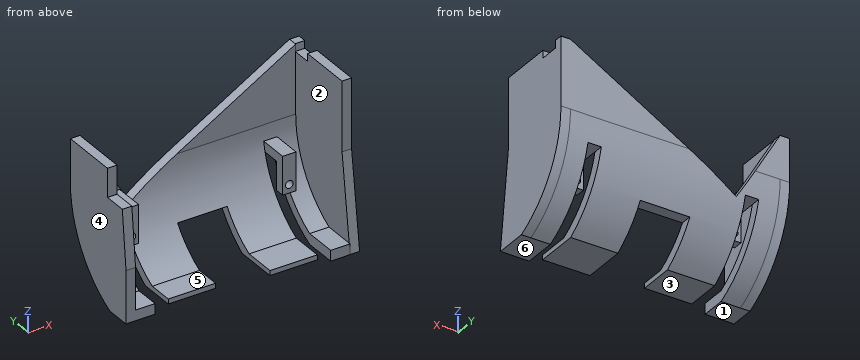
from build123d import *

# Parameters (mm, degrees)
BOSS_EXTRUDE1_DEPTH = 110
CUT_EXTRUDE1_DEPTH  = 110
SKETCH3_W           = 110
SKETCH3_H           = 22.912878475
CUT_EXTRUDE2_DEPTH  = 110
SKETCH4_W           = 10.2
SKETCH4_H           = 5.559027913
SKETCH4_W_2         = 24.8
SKETCH4_H_2         = 2.559027913
BOSS_EXTRUDE2_DEPTH = 13
SKETCH5_W           = 7
SKETCH5_H           = 5
BOSS_EXTRUDE3_DEPTH = 16
SKETCH6_W           = 10.2
SKETCH6_H           = 5.559027913
SKETCH6_W_2         = 24.8
SKETCH6_H_2         = 2.559027913
BOSS_EXTRUDE4_DEPTH = 4
CUT_EXTRUDE3_DEPTH  = 64
SKETCH8_W           = 7
SKETCH8_H           = 5
BOSS_EXTRUDE5_DEPTH = 15
SKETCH9_R           = 2
CUT_EXTRUDE4_DEPTH  = 10
BOSS_EXTRUDE6_START = 5
BOSS_EXTRUDE6_DEPTH = 5
BOSS_EXTRUDE7_DEPTH = 5


with BuildPart() as part:
    # Sketch1 → Boss-Extrude1 (new body)
    with BuildSketch(Plane(origin=(0, 0, 0), x_dir=(0, 0, -1), z_dir=(1, 0, 0))):
        with BuildLine():
            Line((0, 55), (-36, 55))
            Line((-36, 55), (-36, 50))
            Line((-36, 50), (0, 50))
            ThreePointArc((0, 50), (35.355339059, 35.355339059), (50, 0))
            Line((50, 0), (50, -1))
            Line((50, -1), (55, -1))
            Line((55, -1), (55, 0))
            ThreePointArc((55, 0), (38.890872965, 38.890872965), (0, 55))
        make_face()
    extrude(amount=BOSS_EXTRUDE1_DEPTH)

    # Sketch2 → Cut-Extrude1 (cut)
    with BuildSketch(Plane(origin=(0, 55, 0), x_dir=(1, 0, 0), z_dir=(0, 1, 0))):
        Polygon((99.8, 13), (92.8, 13), (92.8, 47), (68, 47), (68, 29), (42, 29), (42, 47), (17.2, 47), (17.2, 13), (10.2, 13), (10.2, 50), (-27.805612869, 50), (-27.805612869, 77.075699265), (114.223867828, 77.075699265), (114.223867828, 50), (99.8, 50), align=None)
    extrude(amount=-CUT_EXTRUDE1_DEPTH, mode=Mode.SUBTRACT)

    # Sketch3 → Cut-Extrude2 (cut)
    with BuildSketch(Plane(origin=(0, 0, -50), x_dir=(-1, 0, 0), z_dir=(0, 0, -1))):
        with Locations((-55, 11.456439238)):
            Rectangle(SKETCH3_W, SKETCH3_H)
    extrude(amount=-CUT_EXTRUDE2_DEPTH, mode=Mode.SUBTRACT)

    # Sketch4 → Boss-Extrude2 (add)
    with BuildSketch(Plane.XZ.offset(-22.912878475)):
        with Locations((104.9, -47.220486044)):
            Rectangle(SKETCH4_W, SKETCH4_H)
        with Locations((80.4, -45.720486044)):
            Rectangle(SKETCH4_W_2, SKETCH4_H_2)
        with Locations((29.6, -45.720486044)):
            Rectangle(SKETCH4_W_2, SKETCH4_H_2)
        with Locations((5.1, -47.220486044)):
            Rectangle(SKETCH4_W, SKETCH4_H)
    extrude(amount=BOSS_EXTRUDE2_DEPTH)

    # Sketch5 → Boss-Extrude3 (add)
    with BuildSketch(Plane.XZ.offset(-50)):
        with Locations((13.7, -10.5)):
            Rectangle(SKETCH5_W, SKETCH5_H)
        with Locations((96.3, -10.5)):
            Rectangle(SKETCH5_W, SKETCH5_H)
    extrude(amount=BOSS_EXTRUDE3_DEPTH)

    # Sketch6 → Boss-Extrude4 (add)
    with BuildSketch(Plane.XZ.offset(-9.912878475)):
        with Locations((104.9, -47.220486044)):
            Rectangle(SKETCH6_W, SKETCH6_H)
        with Locations((80.4, -45.720486044)):
            Rectangle(SKETCH6_W_2, SKETCH6_H_2)
    extrude(amount=BOSS_EXTRUDE4_DEPTH)

    # Sketch7 → Cut-Extrude3 (cut)
    with BuildSketch(Plane(origin=(0, 55, 0), x_dir=(1, 0, 0), z_dir=(0, 1, 0))):
        Polygon((110, -36), (21.665408814, 15), (0, -22.525588833), (0, -36), align=None)
    extrude(amount=-CUT_EXTRUDE3_DEPTH, mode=Mode.SUBTRACT)

    # Sketch8 → Boss-Extrude5 (add)
    with BuildSketch(Plane(origin=(0, 0, -13), x_dir=(-1, 0, 0), z_dir=(0, 0, -1))):
        with Locations((-13.7, 36.5)):
            Rectangle(SKETCH8_W, SKETCH8_H)
        with Locations((-96.3, 36.5)):
            Rectangle(SKETCH8_W, SKETCH8_H)
    extrude(amount=BOSS_EXTRUDE5_DEPTH)

    # Sketch9 → Cut-Extrude4 (cut)
    with BuildSketch(Plane(origin=(0, 39, 0), x_dir=(1, 0, 0), z_dir=(0, 1, 0))):
        with Locations(Location((13.7, 23.6, 0), (0, 0, 270))):
            Circle(SKETCH9_R)
        with Locations(Location((96.3, 23.6, 0), (0, 0, 270))):
            Circle(SKETCH9_R)
    extrude(amount=-CUT_EXTRUDE4_DEPTH, mode=Mode.SUBTRACT)

    # Sketch10 → Boss-Extrude6 (add)
    with BuildSketch(Plane.ZY.offset(BOSS_EXTRUDE6_START)):
        with BuildLine():
            Line((-50, 9.912878475), (-22.474411167, 9.912878475))
            Line((-22.474411167, 9.912878475), (7.525588833, 12.912878475))
            Line((7.525588833, 12.912878475), (7.525588833, 24.912878475))
            Line((7.525588833, 24.912878475), (22.525588833, 24.912878475))
            Line((22.525588833, 24.912878475), (22.525588833, 55))
            Line((22.525588833, 55), (0, 55))
            ThreePointArc((0, 55), (-29.705148408, 46.28827236), (-50, 22.912878475))
            Line((-50, 22.912878475), (-50, 9.912878475))
        make_face()
    extrude(amount=-BOSS_EXTRUDE6_DEPTH)

    # Sketch11 → Boss-Extrude7 (add)
    with BuildSketch(Plane(origin=(110, 0, 0), x_dir=(0, 0, -1), z_dir=(1, 0, 0))):
        with BuildLine():
            Line((-36, 50.412878475), (-32, 50.412878475))
            Line((-32, 50.412878475), (-32, 40.412878475))
            Line((-32, 40.412878475), (-36, 40.412878475))
            Line((-36, 40.412878475), (-36, 12.412878475))
            Line((-36, 12.412878475), (0.424300308, 12.412878475))
            Line((0.424300308, 12.412878475), (50, 5.912878475))
            Line((50, 5.912878475), (50, 22.912878475))
            ThreePointArc((50, 22.912878475), (29.705148408, 46.28827236), (0, 55))
            Line((0, 55), (-36, 55))
            Line((-36, 55), (-36, 50.412878475))
        make_face()
    extrude(amount=BOSS_EXTRUDE7_DEPTH)


solid = part.part
Read the model definition and answer for the solid it produces. Units are mm, in the model's axes. Face numbers are marked on the shaded views. A direction names the side the tool comes from. Give positions to 0.01 mm unless a question says otherwise; leave off trailing zeros. Write each loop counter-clockwise with the first axis right and the second up, starting at its lowest first coordinate (ties: lowest second). Pieces come first, ordered by that corner, then holes. Notation, with made-up numbers: (75.25, 73.25) - (86.25, 73.25) arc R27 ccw to (86.25, 103.25) - close; hole circle Ø10 at (71.25, -10.75). An arc over 180 degrees is marked (long way). Return JSON: item names as keys, results as strings.
Q1. For the marked faces 1, 2 and 3, determine the directions among +Z, -Z, +X, -X, +Y, -Y from which every point of the face is accessible in a straight line to the end or side of a thin tool.
Reply:
{"face 1": "-Z, +X, -X, +Y, -Y", "face 2": "+Z, -Y", "face 3": "-Z, +Y, -Y"}
Q2. A cutting plane is placed at D-D, the plane z = -41.5. Determine the outline of the cut face in (x, y).
Reply:
{"outline": "(-5, 9.91) - (0, 9.91) - (0, 27.89) - (10.2, 27.89) - (10.2, 36.09) - (-5, 36.09) - close; (17.2, 27.89) - (42, 27.89) - (42, 36.09) - (17.2, 36.09) - close; (68, 27.89) - (92.8, 27.89) - (92.8, 36.09) - (68, 36.09) - close; (99.8, 27.89) - (110, 27.89) - (110, 7.03) - (115, 7.03) - (115, 36.09) - (99.8, 36.09) - close"}
Q3. A cutting plane is placed at B-B, the plane z = -9.5. Determine the outline of the cut face in (x, y).
Reply:
{"outline": "(-5, 11.21) - (0, 11.21) - (0, 49.09) - (10.2, 49.09) - (10.2, 34) - (17.2, 34) - (17.2, 49.09) - (18.49, 49.09) - (18.49, 54.17) - (-5, 54.17) - close; (31.19, 49.09) - (92.8, 49.09) - (92.8, 34) - (99.8, 34) - (99.8, 49.09) - (110, 49.09) - (110, 11.22) - (115, 11.22) - (115, 54.17) - (31.19, 54.17) - close"}
Q4. For a pull along X with two mould halves and no side action, classify the marked faces 4, 5 and 6 as released by +X, released by -X, zero draft, split by the parting line, or undercut.
Reply:
{"face 4": "released by -X", "face 5": "undercut", "face 6": "zero draft"}
Q5. Given P1, Ø6, axis at x = 57, z = 11.5, coming from the -Y side; P2, Ø20.5, axis at x = 33, y = 15.5, coming from the -Z side; P3, Ø1.5, axis at x = 97, y = 37.5, coming from the -Z side; P4, Ø2, axis at x = 97.5, z = -22, coming from the +Y side, each flat-ended and moving along its own axis, determine where each tip first touches the part or whether it passes through.
Reply:
{"P1": "through", "P2": "z = -47", "P3": "z = -28", "P4": "y = 39"}
Q6. Consider line 1 along X through (y, z) = (37, -11); line 2 along X through (y, z) = (36.8, -23.6); line 3 along X through (y, z) = (48.5, 20.5). Determine where each line is inside the solid, lowest interval first. Write a range as [from, to].
Reply:
{"line 1": "[-5, 0], [10.2, 17.2], [92.8, 99.8], [110, 115]", "line 2": "[-5, 0], [10.2, 11.7], [15.7, 17.2], [92.8, 94.3], [98.3, 99.8], [110, 115]", "line 3": "[-5, 0], [110, 115]"}
Q7. A cutting plane is placed at A-A, the plane y = 17. Determine the outline of the cut face in (x, z).
Reply:
{"outline": "(-5, -50) - (10.2, -50) - (10.2, -44.44) - (0, -44.44) - (0, 7.53) - (-5, 7.53) - close; (17.2, -47) - (42, -47) - (42, -44.44) - (17.2, -44.44) - close; (68, -47) - (92.8, -47) - (92.8, -44.44) - (68, -44.44) - close; (99.8, -50) - (115, -50) - (115, 36) - (110, 36) - (110, -44.44) - (99.8, -44.44) - close"}
Q8. A cutting plane is placed at C-C, the plane y = 42. Determine the outline of the cut face in (x, z), and give its area (3 significant figures).
Reply:
{"outline": "(-5, -35.51) - (10.2, -35.51) - (10.2, -27.13) - (0, -27.13) - (0, 22.53) - (-5, 22.53) - close; (10.2, -13) - (17.2, -13) - (17.2, -8) - (10.2, -8) - close; (17.2, -35.51) - (42, -35.51) - (42, -29) - (68, -29) - (68, -35.51) - (92.8, -35.51) - (92.8, -27.13) - (17.2, -27.13) - close; (92.8, -13) - (99.8, -13) - (99.8, -8) - (92.8, -8) - close; (99.8, -35.51) - (115, -35.51) - (115, 32) - (110, 32) - (110, -27.13) - (99.8, -27.13) - close", "area": "1,330 mm²"}
